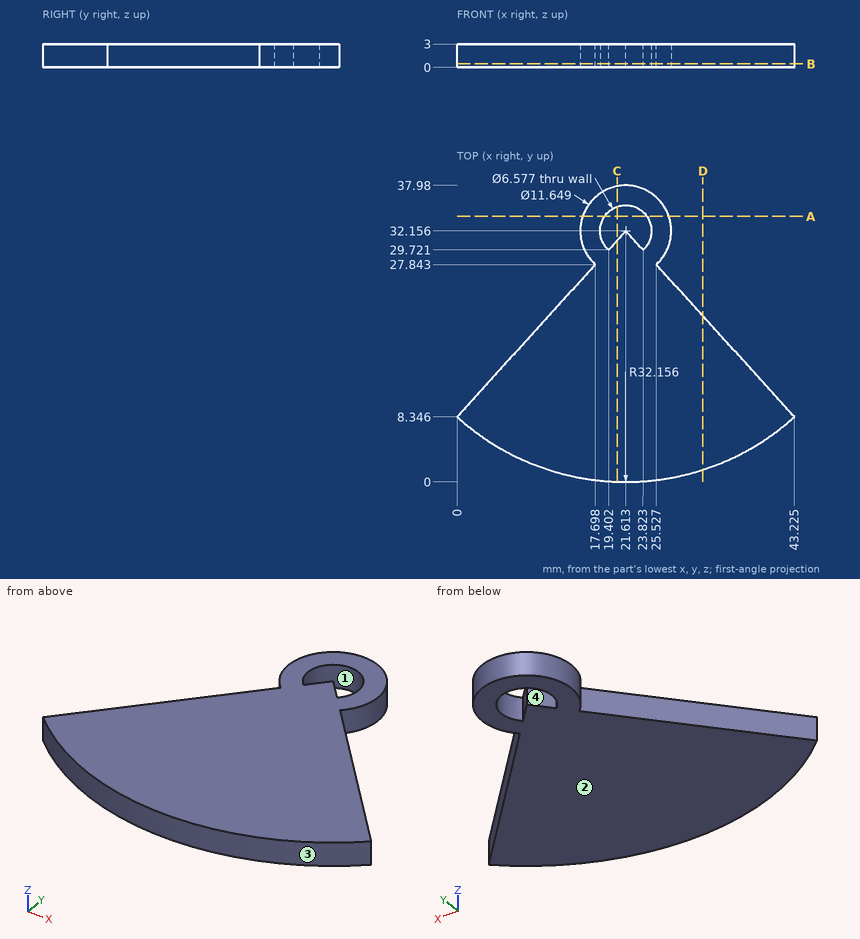
Job drawing, mm, ordinate dimensions from the low corner. One solid piece. Round coordinates to 2 decimals unless told otherwise and drop trailing zeros. Write each loop counter-clockwise with the first axis right and the second up, starting at its lowest first coordinate (ties: lowest second). Pieces come first, ordered by that corner, then holes.
1) Mould opens along X. For the marked faces 1, 2, 3 and 4 say: +X half, -X half, draft (parallel to the pull), parting line (faces both ways), or undercut.
2) Band-saw the part on C-C, the plane x = 20.5. List the corners of the cut face in (y, z), and give its area (3 significant figures).
3) Band-saw the part on A-A, the plane y = 34. List the corners of the cut face in (x, z) (1 decimal).
4) Drill centre lines: probe 1 along X at (y, z) = (34.5, 0.55) (1 decimal); probe 2 along X at (y, z) = (34, 2.1) (1 decimal); probe 3 along Y at (x, z) = (15.5, 1.4) (1 decimal). Where is each one in solid material? Low to high.
5) Band-saw the part on B-B, the plane z = 0.45. List the corners of the cut face in (x, y) (1 decimal).
6) Band-saw the part on D-D, the plane x = 31.5. List the corners of the cut face in (y, z).
7) Pin check, flat tip, straight feed: pin 1 (1 mm diameter, centred on x = 25.5, z = 2.5, fed in from -Y). Stop position of the tip, or through.
Ans:
1. face 1: undercut
1. face 2: draft
1. face 3: parting line
1. face 4: undercut
2. outline: (0.02, 0) - (30.93, 0) - (30.93, 3) - (0.02, 3) - close; (35.25, 0) - (37.87, 0) - (37.87, 3) - (35.25, 3) - close
2. area: 101 mm2
3. outline: (16.1, 0) - (18.9, 0) - (18.9, 3) - (16.1, 3) - close; (24.3, 0) - (27.1, 0) - (27.1, 3) - (24.3, 3) - close
4. probe 1: x = 16.3 to 19.3, 23.9 to 26.9
4. probe 2: x = 16.1 to 18.9, 24.3 to 27.1
4. probe 3: y = 0.6 to 25.4
5. outline: (0, 8.3) arc R32.2 ccw to (43.2, 8.3) - (25.5, 27.8) arc R5.8 ccw (long way) to (17.7, 27.8) - close; hole (19.4, 29.7) - (21.6, 32.2) - (23.8, 29.7) arc R3.3 ccw (long way) to start
6. outline: (1.56, 0) - (21.26, 0) - (21.26, 3) - (1.56, 3) - close
7. pin 1: stops at y = 0.18
